Can you work these out from the model? Positions are in its coordinate system, mm. Face numbers are marked on the shaded views. A direction names the side the tool comes from. Coordinates: 2 decimals unless noted, no trailing zeros. Order: outer loops, then holes, each group sorted by start corner. A loop starts at its lowest first (then second) coordinate and runs counter-clockwise, first axis right, second up. Notation, with made-up numbers: (30, 7.5) -> (37, 7.5) arc R8 ccw to (37, 21.5) -> close; hole circle Ø4 at (6.25, 16). An arc over 180 degrees is marked (long way). Answer in a Markdown table with one row per item. Add a question column.
1. Imagine slicing it at A-A on y = -38. Write out the boundary of the cut face in (x, z), plus the area to 3 significant figures.
2. On a 3-axis mill with a long thin cutter (end or side, diameter ignored), from which of +Z, -Z, +X, -X, +Y, -Y can I reach the whole of each face in a straight line? I mean the marked faces 3 and 4. Say none if no direction works.
3. If I drill on line 1 along X through (y, z) = (-35, 0); line 2 along X through (y, z) = (-8.5, 0); line 3 along Z through (x, y) = (0.25, -38), over which ranges is the centre line in solid material (lowest first)? Write a range as [from, to].
4. We'd pull the mould along Z, two halves only. Please class the marked faces 1 and 2: pulls with the +Z half, pulls with the -Z half, needs draft (parallel to the pull), parting line crosses it, or undercut.
5. Imagine slicing it at B-B on y = -25. Write out the boundary of the cut face in (x, z), plus the area to 3 significant figures.
6. Will these pins go through, and if not, where does the flat tip stop? pin 1 (0.8 mm diameter, centred on x = 0.5, z = -6, fed in from -Y); pin 2 (8 mm diameter, centred on x = -4, z = 2.5, fed in from +Y); pin 3 (3 mm diameter, centred on x = 0.5, y = -5.5, fed in from -Z); pin 4 (3.5 mm diameter, centred on x = 4, z = -3.5, fed in from -Y).
from build123d import *

# Parameters (mm, degrees)
PER_AGE_T_TE_D           = 12
PER_AGE_T_TE_DEPTH       = 20
PER_AGE_T_TE_CSINK_D     = 15
PER_AGE_T_TE_CSINK_ANGLE = 90
PER_AGE_T_TE_TIP         = 3.605163714
H_XAGONE_DEPTH           = 12
CENTRAGE_D               = 3
CENTRAGE_DEPTH           = 6
CENTRAGE_CSINK_D         = 5
CENTRAGE_CSINK_ANGLE     = 60
CENTRAGE_TIP             = 0.901290929
PER_AGE_AXE_D            = 12
PER_AGE_AXE_DEPTH        = 12
PER_AGE_AXE_CSINK_D      = 13
PER_AGE_AXE_CSINK_ANGLE  = 90
PER_AGE_AXE_TIP          = 3.605163714
ESQUISSE9_W              = 7
ESQUISSE9_H              = 8.5
ESQUISSE9_W_2            = 1.5
ESQUISSE9_H_2            = 2
ESQUISSE10_W             = 2
ESQUISSE10_H             = 8.5
CHANFREIN1_SIZE          = 1.5


with BuildPart() as part:
    # Esquisse1 → Base-Révolution (revolve)
    with BuildSketch(Plane.XY, mode=Mode.PRIVATE) as base_r_volution_sk:
        with BuildLine():
            Line((0, 0), (7.680127019, 0))
            Line((7.680127019, 0), (8.35, -2.5))
            Line((8.35, -2.5), (8.35, -8))
            Line((8.35, -8), (8.49, -8.14))
            Line((8.49, -8.14), (8.49, -19.14))
            Line((8.49, -19.14), (8.21, -19.42))
            Line((8.21, -19.42), (8.21, -21.24))
            ThreePointArc((8.21, -21.24), (8.327157288, -21.522842712), (8.61, -21.64))
            Line((8.61, -21.64), (8.99, -21.64))
            Line((8.99, -21.64), (9.49, -21.14))
            Line((9.49, -21.14), (10, -21.14))
            Line((10, -21.14), (12, -23.14))
            Line((12, -23.14), (12, -40.64))
            Line((12, -40.64), (10, -42.64))
            Line((10, -42.64), (10, -43.14))
            ThreePointArc((10, -43.14), (10.292893219, -43.847106781), (11, -44.14))
            Line((11, -44.14), (19, -44.14))
            Line((19, -44.14), (19, -45.14))
            Line((19, -45.14), (12.07179677, -49.14))
            Line((12.07179677, -49.14), (0, -49.14))
            Line((0, -49.14), (0, 0))
        make_face()
    revolve(base_r_volution_sk.sketch.rotate(Axis((0, -10, 0), (0, -1, 0)), 90), axis=Axis((0, -10, 0), (0, -1, 0)))

    # Perçage tête
    with Locations(Plane.XZ.offset(49.14)):
        with Locations((0, 0)):
            CounterSinkHole(PER_AGE_T_TE_D / 2, PER_AGE_T_TE_CSINK_D / 2, depth=PER_AGE_T_TE_DEPTH, counter_sink_angle=PER_AGE_T_TE_CSINK_ANGLE)
            with Locations((0, 0, -(PER_AGE_T_TE_DEPTH + PER_AGE_T_TE_TIP / 2))):  # 118° drill point
                Cone(0, PER_AGE_T_TE_D / 2, PER_AGE_T_TE_TIP, mode=Mode.SUBTRACT)

    # Esquisse4 → Héxagone (cut)
    with BuildSketch(Plane.XZ.offset(49.14)):
        with BuildLine():
            Line((-0.25, 6.783865663), (-5.75, 3.608439182))
            ThreePointArc((-5.75, 3.608439182), (-5.933012702, 3.425426481), (-6, 3.175426481))
            Line((-6, 3.175426481), (-6, -3.175426481))
            ThreePointArc((-6, -3.175426481), (-5.933012702, -3.425426481), (-5.75, -3.608439182))
            Line((-5.75, -3.608439182), (-0.25, -6.783865663))
            ThreePointArc((-0.25, -6.783865663), (0, -6.850852961), (0.25, -6.783865663))
            Line((0.25, -6.783865663), (5.75, -3.608439182))
            ThreePointArc((5.75, -3.608439182), (5.933012702, -3.425426481), (6, -3.175426481))
            Line((6, -3.175426481), (6, 3.175426481))
            ThreePointArc((6, 3.175426481), (5.933012702, 3.425426481), (5.75, 3.608439182))
            Line((5.75, 3.608439182), (0.25, 6.783865663))
            ThreePointArc((0.25, 6.783865663), (0, 6.850852961), (-0.25, 6.783865663))
        make_face()
    extrude(amount=-H_XAGONE_DEPTH, mode=Mode.SUBTRACT)

    # Centrage
    with Locations(Plane(origin=(0, 0, 0), x_dir=(-1, 0, 0), z_dir=(0, 1, 0))):
        with Locations((0, 0)):
            CounterSinkHole(CENTRAGE_D / 2, CENTRAGE_CSINK_D / 2, depth=CENTRAGE_DEPTH, counter_sink_angle=CENTRAGE_CSINK_ANGLE)
            with Locations((0, 0, -(CENTRAGE_DEPTH + CENTRAGE_TIP / 2))):  # 118° drill point
                Cone(0, CENTRAGE_D / 2, CENTRAGE_TIP, mode=Mode.SUBTRACT)

    # Perçage axe
    with Locations(Plane(origin=(0, 0, 0), x_dir=(-1, 0, 0), z_dir=(0, 1, 0))):
        with Locations((0, 0)):
            CounterSinkHole(PER_AGE_AXE_D / 2, PER_AGE_AXE_CSINK_D / 2, depth=PER_AGE_AXE_DEPTH, counter_sink_angle=PER_AGE_AXE_CSINK_ANGLE)
            with Locations((0, 0, -(PER_AGE_AXE_DEPTH + PER_AGE_AXE_TIP / 2))):  # 118° drill point
                Cone(0, PER_AGE_AXE_D / 2, PER_AGE_AXE_TIP, mode=Mode.SUBTRACT)

    # Esquisse9 → Enlèvement tête (revolve, cut)
    with BuildSketch(Plane.XY, mode=Mode.PRIVATE) as enl_vement_t_te_sk:
        with Locations((15.5, -44.89)):
            Rectangle(ESQUISSE9_W, ESQUISSE9_H)
        with Locations((11.25, -22.14)):
            Rectangle(ESQUISSE9_W_2, ESQUISSE9_H_2)
    revolve(enl_vement_t_te_sk.sketch.rotate(Axis((0, -50, 0), (0, 1, 0)), 90), axis=Axis((0, -50, 0), (0, 1, 0)), mode=Mode.SUBTRACT)

    # Esquisse10 → Suppression gorge (revolve)
    with BuildSketch(Plane.XY, mode=Mode.PRIVATE) as suppression_gorge_sk:
        with Locations((11, -44.89)):
            Rectangle(ESQUISSE10_W, ESQUISSE10_H)
    revolve(suppression_gorge_sk.sketch.rotate(Axis((0, -47.996933622, 0), (0, 1, 0)), 90), axis=Axis((0, -47.996933622, 0), (0, 1, 0)))

    # Chanfrein1
    chanfrein1_edges = [part.edges().sort_by_distance(p)[0] for p in [
        (0, -49.14, 12),
    ]]
    chamfer(chanfrein1_edges, length=CHANFREIN1_SIZE)


solid = part.part
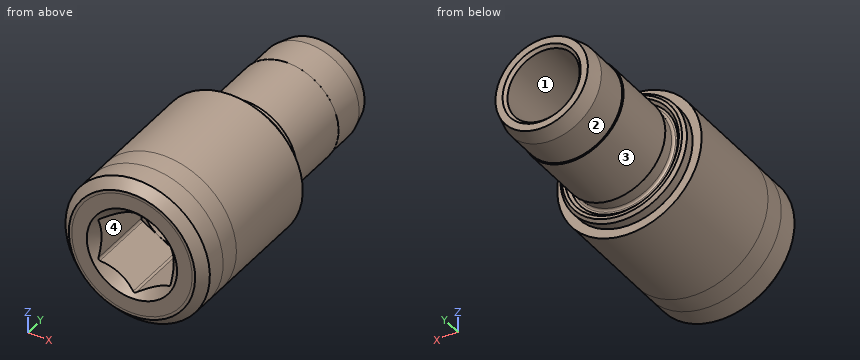
Answers follow:
| question | item | result |
|---|---|---|
| 1 | outline | circle Ø24 at (0, 0); hole (-6, -3.18) arc R0.5 ccw to (-5.75, -3.61) -> (-0.25, -6.78) arc R0.5 ccw to (0.25, -6.78) -> (5.75, -3.61) arc R0.5 ccw to (6, -3.18) -> (6, 3.18) arc R0.5 ccw to (5.75, 3.61) -> (0.25, 6.78) arc R0.5 ccw to (-0.25, 6.78) -> (-5.75, 3.61) arc R0.5 ccw to (-6, 3.18) -> close |
| 1 | area | 328 mm² |
| 2 | face 3 | +Y |
| 2 | face 4 | -Y |
| 3 | line 1 | x = [-12, -6], [6, 12] |
| 3 | line 2 | x = [-8.49, -6], [6, 8.49] |
| 3 | line 3 | z = [-12, -6.78], [6.78, 12] |
| 4 | face 1 | undercut |
| 4 | face 2 | parting line crosses it |
| 5 | outline | circle Ø24 at (0, 0) |
| 5 | area | 452 mm² |
| 6 | pin 1 | stops at y = -37.14 |
| 6 | pin 2 | stops at y = 0 |
| 6 | pin 3 | stops at z = -8.35 |
| 6 | pin 4 | stops at y = -48.71 |
